Autodesk Inventor part; units mm, degrees
ref_plane "YZ Plane" through (0, 0, 0) normal (1, 0, 0) x (0, 1, 0)
ref_plane "XZ Plane" through (0, 0, 0) normal (0, 1, 0) x (-1, 0, 0)
ref_plane "XY Plane" through (0, 0, 0) normal (0, 0, 1) x (1, 0, 0)
sketch "Sketch1" plane through (0, 0, 0) normal (0, 1, 0) x (-1, 0, 0)
  line L0 (0, 0) -> (98.806, 0)
  line L1 (98.806, 0) -> (98.806, -8)
  line L2 (98.806, -8) -> (0, -8)
  line L3 (0, -8) -> (0, 0)
  line L4 (0, -8) -> (-4, -8)
  line L5 (-4, -8) -> (-4, 0)
  line L6 (-4, 0) -> (0, 0)
  line L7 (0, 0) -> (0, -8)
  line L8 (98.806, 0) -> (108.806, 0)
  line L9 (108.806, 0) -> (108.806, -8)
  line L10 (108.806, -8) -> (98.806, -8)
  point P0 (0, 0)
  dimension "d0" = 98.806
  dimension "d1" = 8
  dimension "d2" = 4
  dimension "d3" = 8
  dimension "d4" = 10
extrude "Extrusion1" add sketch "Sketch1" along normal blind 30 contours L3 L4 L5 L6
extrude "Extrusion2" add sketch "Sketch1" along normal blind 4 contours L0 L1 L2 L3 | L8 L9 L10 L1
sketch "Sketch2" plane through (0, 4, 0) normal (0, 1, 0) x (1, 0, 0)
  line L0 (-108.806, 8) -> (-108.806, 0)
  line L1 (-108.806, 4) -> (-103.806, 4)
  point P0 (0, 0)
  dimension "d9" = 5
hole "Hole1" at (-103.806, 4, -4) direction (0, -1, 0) diameter 3.4 end through all
sketch "Sketch3" plane through (-108.806, 0, -8) normal (-1, 0, 0) x (0, 0, 1)
  line L0 (0, 4) -> (8, 4)
  line L1 (0, 4) -> (8, 4)
  line L2 (8, 4) -> (8, 2)
  line L3 (8, 2) -> (0, 2)
  line L4 (0, 2) -> (0, 4)
  point P0 (8, 0)
  point P1 (8, 4)
  dimension "d17" = 8
  dimension "d18" = 2
extrude "Extrusion3" cut sketch "Sketch3" against normal blind 10
sketch "Sketch4" plane through (-108.806, 0, -8) normal (-1, 0, 0) x (0, 0, 1)
  line L0 (8, 2) -> (0, 2)
  line L1 (0, 0) -> (0, 2)
  line L2 (0, 0) -> (8, 0)
  line L3 (8, 0) -> (8, 2)
extrude "Extrusion4" add sketch "Sketch4" along normal blind 2.54
properties part number "brace2"
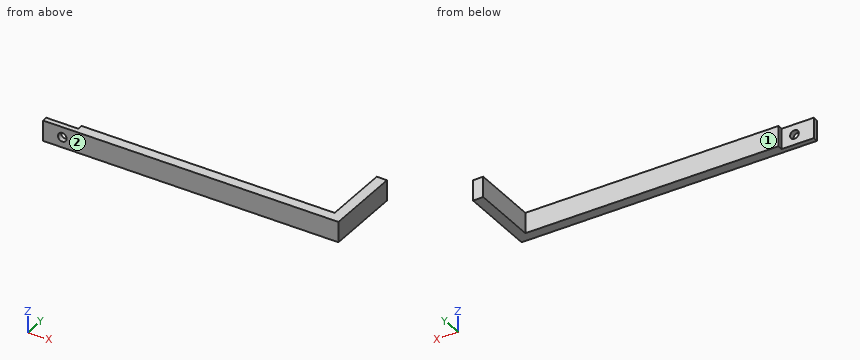
Here's how the part is built. I have some questions about the finished solid (model axes, mm). Face numbers are marked on the shaded views. A direction names the side the tool comes from. Coordinates: 2 decimals unless noted, no trailing zeros. Write each loop counter-clockwise with the first axis right and the second up, starting at its lowest first coordinate (ties: lowest second). Pieces come first, ordered by that corner, then holes. Notation, with made-up numbers: (40, 30.5) - (82, 30.5) arc R21 ccw to (82, 67.5) - close; hole circle Ø7 at (-17.75, 71). An arc over 180 degrees is marked (long way). One line per item, written item: value.
1) Suppose I cut it at B-B on x = -84. Write out the boundary of the cut face in (y, z), and give its area (3 significant figures).
Model answer:
outline: (0, -8) - (4, -8) - (4, 0) - (0, 0) - close
area: 32.0 mm²
2) Suppose I cut it at A-A on z = -4. Write out the boundary of the cut face in (x, y).
Model answer:
outline: (-111.35, 0) - (-105.51, 0) - (-105.51, 2) - (-111.35, 2) - close; (-102.11, 0) - (4, 0) - (4, 30) - (0, 30) - (0, 4) - (-98.81, 4) - (-98.81, 2) - (-102.11, 2) - close
3) I need wall thicknesses on line 1 along X through (y, z) = (0.55, -4); line 2 along X through (y, z) = (20, -5.25); line 3 along Y through (x, z) = (-101.5, -6). Which ranges of each line are inside material? Lowest first, please.
Model answer:
line 1: x = -111.35 to -105.51, -102.11 to 4
line 2: x = 0 to 4
line 3: y = 0 to 2
4) On a 3-axis mill with a long thin cutter (end or side, diameter ignored), from which of +Z, -Z, +X, -X, +Y, -Y can I reach the whole of each face in a straight line? I mean the marked faces 1 and 2. Say none if no direction works.
Model answer:
face 1: +Z, -Z, -X, +Y
face 2: +Z, -Z, +X, -X, -Y
5) I'm going to push flat-ended pins straight in: P1, Ø2.5, axis at x = -103, z = -5.5, coming from the +Y side; P2, Ø8, axis at x = -27, y = 9.5, coming from the +Z side; P3, Ø10, axis at x = -74, y = 6.5, coming from the +Z side; P4, Ø1.5, axis at y = 24.5, z = -2, coming from the -X side. Where does each tip first touch, or does it pass through?
Model answer:
P1: stops at y = 2
P2: passes through
P3: stops at z = 0
P4: stops at x = 0
